For this review, take the finished solid that the model builds, in its own axes (mm). Face numbers are marked on the shaded views. A direction names the side the tool comes from. Round coordinates to 2 decimals unless told otherwise and drop trailing zeros. Write each loop counter-clockwise with the first axis right and the second up, starting at its lowest first coordinate (ties: lowest second). Pieces come first, ordered by that corner, then holes.
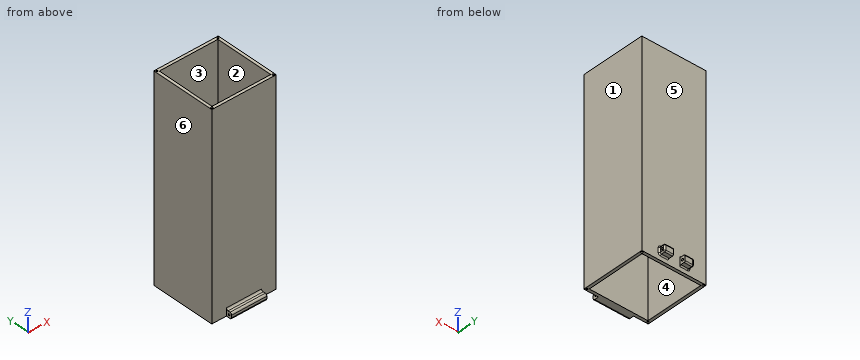
from build123d import *

# Parameters (mm, degrees)
SKETCH1_W                = 110
SKETCH1_H                = 110
SKETCH1_W_2              = 100.2
SKETCH1_H_2              = 100.2
BOSS_EXTRUDE1_DEPTH      = 340.5
CUT_EXTRUDE1_REACH       = 351.271
SKETCH2_R                = 1.575
BOSS_EXTRUDE3_DEPTH      = 30
BOSS_EXTRUDE3_DEPTH_BACK = 30
SKETCH3_W                = 10
SKETCH3_H                = 10
SKETCH4_R                = 1.5
CUT_EXTRUDE2_DEPTH       = 60
SKETCH6_W                = 15
SKETCH6_H                = 12
BOSS_EXTRUDE4_DEPTH      = 10
CUT_EXTRUDE3_REACH       = 357.76
SKETCH7_R                = 2
FILLET1_R                = 2
FILLET2_R                = 3


with BuildPart() as part:
    # Sketch1 → Boss-Extrude1 (new body)
    with BuildSketch(Plane.XY):
        Rectangle(SKETCH1_W, SKETCH1_H)
        Rectangle(SKETCH1_W_2, SKETCH1_H_2, mode=Mode.SUBTRACT)
    extrude(amount=BOSS_EXTRUDE1_DEPTH)

    # Sketch2 → Cut-Extrude1 (cut, up to next)
    with BuildSketch(Plane.XY.offset(340.5), mode=Mode.PRIVATE) as cut_extrude1_sk1:
        with Locations((-52.149125113, 52.149125113)):
            Circle(SKETCH2_R)
    cut_extrude1_tool1 = extrude(cut_extrude1_sk1.sketch, amount=-CUT_EXTRUDE1_REACH, mode=Mode.PRIVATE) & part.part
    # Sketch2 → Cut-Extrude1 (cut, up to next)
    with BuildSketch(Plane.XY.offset(340.5), mode=Mode.PRIVATE) as cut_extrude1_sk2:
        with Locations((52.149125113, 52.149125113)):
            Circle(SKETCH2_R)
    cut_extrude1_tool2 = extrude(cut_extrude1_sk2.sketch, amount=-CUT_EXTRUDE1_REACH, mode=Mode.PRIVATE) & part.part
    # Sketch2 → Cut-Extrude1 (cut, up to next)
    with BuildSketch(Plane.XY.offset(340.5), mode=Mode.PRIVATE) as cut_extrude1_sk3:
        with Locations((52.149125113, -52.149125113)):
            Circle(SKETCH2_R)
    cut_extrude1_tool3 = extrude(cut_extrude1_sk3.sketch, amount=-CUT_EXTRUDE1_REACH, mode=Mode.PRIVATE) & part.part
    # Sketch2 → Cut-Extrude1 (cut, up to next)
    with BuildSketch(Plane.XY.offset(340.5), mode=Mode.PRIVATE) as cut_extrude1_sk4:
        with Locations((-52.149125113, -52.149125113)):
            Circle(SKETCH2_R)
    cut_extrude1_tool4 = extrude(cut_extrude1_sk4.sketch, amount=-CUT_EXTRUDE1_REACH, mode=Mode.PRIVATE) & part.part
    add(cut_extrude1_tool1.solids().sort_by_distance((-52.149125, 52.149125, 340.5))[0], mode=Mode.SUBTRACT)
    add(cut_extrude1_tool2.solids().sort_by_distance((52.149125, 52.149125, 340.5))[0], mode=Mode.SUBTRACT)
    add(cut_extrude1_tool3.solids().sort_by_distance((52.149125, -52.149125, 340.5))[0], mode=Mode.SUBTRACT)
    add(cut_extrude1_tool4.solids().sort_by_distance((-52.149125, -52.149125, 340.5))[0], mode=Mode.SUBTRACT)

    # Sketch3 → Boss-Extrude3 (add, two sides: drawn at the far end of the back side and taken through both)
    with BuildSketch(Plane(origin=(0, 0, 0), x_dir=(0, 0, -1), z_dir=(1, 0, 0)).offset(-BOSS_EXTRUDE3_DEPTH_BACK)):
        with Locations((-5, -60)):
            Rectangle(SKETCH3_W, SKETCH3_H)
    extrude(amount=BOSS_EXTRUDE3_DEPTH + BOSS_EXTRUDE3_DEPTH_BACK)

    # Sketch4 → Cut-Extrude2 (cut)
    with BuildSketch(Plane.ZY.offset(30)):
        with Locations((5, -60)):
            Circle(SKETCH4_R)
    extrude(amount=-CUT_EXTRUDE2_DEPTH, mode=Mode.SUBTRACT)

    # Sketch6 → Boss-Extrude4 (add)
    with BuildSketch(Plane(origin=(0, 55, 0), x_dir=(1, 0, 0), z_dir=(0, 1, 0))):
        with Locations((-17.5, -15)):
            Rectangle(SKETCH6_W, SKETCH6_H)
        with Locations((17.5, -15)):
            Rectangle(SKETCH6_W, SKETCH6_H)
    extrude(amount=BOSS_EXTRUDE4_DEPTH)

    # Cut-Extrude3: up to this face of the body (flat: up to its plane)
    cut_extrude3_end = Plane(part.part.faces().sort_by_distance((25, 60, 15))[0])
    # Sketch7 → Cut-Extrude3 (cut, up to the picked face)
    with BuildSketch(Plane.ZY.offset(25), mode=Mode.PRIVATE) as cut_extrude3_sk1:
        with Locations(Location((15, 60, 0), (0, 0, 270))):
            Circle(SKETCH7_R)
    cut_extrude3_tool1 = split(extrude(cut_extrude3_sk1.sketch, amount=-CUT_EXTRUDE3_REACH, mode=Mode.PRIVATE), bisect_by=cut_extrude3_end, keep=Keep.BOTH, mode=Mode.PRIVATE)
    add(cut_extrude3_tool1.solids().sort_by(Axis((-25, 60, 15), (1, 0, 0)))[0], mode=Mode.SUBTRACT)

    # Fillet1
    fillet1_edges = [part.edges().sort_by_distance(p)[0] for p in [
        (-25, 55, 15),
        (-25, 60, 9),
        (-17.5, 55, 21),
        (-25, 60, 21),
        (-17.5, 55, 9),
        (-25, 65, 15),
        (-17.5, 65, 21),
        (-17.5, 65, 9),
        (17.5, 55, 21),
        (25, 55, 15),
        (25, 60, 21),
        (17.5, 55, 9),
        (25, 60, 9),
        (17.5, 65, 21),
        (25, 65, 15),
        (17.5, 65, 9),
    ]]
    fillet(fillet1_edges, radius=FILLET1_R)

    # Fillet2
    fillet2_edges = [part.edges().sort_by_distance(p)[0] for p in [
        (0, -65, 0),
        (0, -65, 10),
        (0, -55, 10),
    ]]
    fillet(fillet2_edges, radius=FILLET2_R)


solid = part.part
(1) For line 1 along Y through (x, z) = (48, 271.5); line 2 along Z through (x, y) = (13, 60), list the stretches that pass through material, from the lowest coordinate up.
Geometry check:
line 1: y = -55 to -50.1, 50.1 to 55
line 2: z = 9 to 13, 17 to 21
(2) We need section B-B, the plane z = 200.5. Give the boundary of the cut face in (x, y) (3 decimals), and give its area (3 significant figures).
Geometry check:
outline: (-55, -55) - (55, -55) - (55, 55) - (-55, 55) - close; hole circle Ø3.15 at (-52.149, -52.149); hole circle Ø3.15 at (-52.149, 52.149); hole (-50.1, -50.1) - (50.1, -50.1) - (50.1, 50.1) - (-50.1, 50.1) - close; hole circle Ø3.15 at (52.149, -52.149); hole circle Ø3.15 at (52.149, 52.149)
area: 2,030 mm2
(3) For the marked faces 1 and 2, list the 3-axis set-ups (+Z, -Z, +X, -X, +Y, -Y) from which the entire face can be reached by the end or side of a thin tool; tool diameter is ignored.
Geometry check:
face 1: +Z, -Z, +X, +Y, -Y
face 2: +Z, -Z
(4) We need section A-A, the plane y = -27.5. Give the boundary of the cut face in (x, z), and give its area (3 significant figures).
Geometry check:
outline: (-55, 0) - (-50.1, 0) - (-50.1, 340.5) - (-55, 340.5) - close; (50.1, 0) - (55, 0) - (55, 340.5) - (50.1, 340.5) - close
area: 3,340 mm2
(5) For pin 1 Ø6.5 at (x, y) = (-19.5, 59) entering from +Z; pin 2 Ø1.5 at (x, z) = (26.5, 117) entering from -Y; pin 3 Ø4.5 at (y, z) = (60, 15) entering from +X, all flat-tipped, find the tip position at first contact; note any pin that passes through.
Geometry check:
pin 1: stops at z = 21.44
pin 2: stops at y = -55
pin 3: stops at x = 25
(6) Mouldability with a two-part tool opening along Y and no side actions: class the marked faces 3, 4, 5 and 6 as pulls with the +Y half, pulls with the -Y half, needs draft (parallel to the pull), parting line crosses it, or undercut.
Geometry check:
face 3: undercut
face 4: undercut
face 5: pulls with the +Y half
face 6: needs draft
